```python
from build123d import *

# Parameters (mm, degrees)
F0_R     = 4.75
F1_DEPTH = 7.5
F2_R     = 50
F3_SIZE  = 1
F5_DEPTH = 25
F6_SIZE  = 1


with BuildPart() as f1:
    # F0 (on Top) → F1 (new body, symmetric)
    with BuildSketch(Plane.XY):
        with BuildLine():
            Line((25, 0), (8.288939, 39.506208))
            ThreePointArc((8.288939, 39.506208), (0, 45), (-8.288939, 39.506208))
            Line((-8.288939, 39.506208), (-25, 0))
            Line((-25, 0), (-8.288939, -39.506208))
            ThreePointArc((-8.288939, -39.506208), (0, -45), (8.288939, -39.506208))
            Line((8.288939, -39.506208), (25, 0))
        make_face()
        with Locations((0, -36)):
            Circle(F0_R, mode=Mode.SUBTRACT)
        with Locations((0, 36)):
            Circle(F0_R, mode=Mode.SUBTRACT)
    extrude(amount=F1_DEPTH, both=True)

    # F2
    f2_edges = [f1.edges().sort_by_distance(p)[0] for p in [
        (-25, 0, 0),
        (25, 0, 0),
    ]]
    fillet(f2_edges, radius=F2_R)

    # F3
    f3_edges = [f1.edges().sort_by_distance(p)[0] for p in [
        (0, 45, 7.5),
        (0, 45, -7.5),
        (-12.524692, -29.492569, 7.5),
        (-12.524692, -29.492569, -7.5),
    ]]
    chamfer(f3_edges, length=F3_SIZE)

    # F4 (on face) → F5 (cut)
    with BuildSketch(Plane.XY.offset(7.5)):
        Polygon((-4.025, 6.971505), (-8.05, 0), (-4.025, -6.971505), (4.025, -6.971505), (8.05, 0), (4.025, 6.971505), align=None)
    extrude(amount=-F5_DEPTH, mode=Mode.SUBTRACT)

    # F6
    f6_edges = [f1.edges().sort_by_distance(p)[0] for p in [
        (-4.75, 36, 7.5),
        (-4.75, 36, -7.5),
        (-4.75, -36, 7.5),
        (-4.75, -36, -7.5),
        (0, -6.971505, 7.5),
        (-6.0375, -3.485752, 7.5),
        (-6.0375, 3.485752, 7.5),
        (0, 6.971505, 7.5),
        (6.0375, 3.485752, 7.5),
        (6.0375, -3.485752, 7.5),
        (0, -6.971505, -7.5),
        (6.0375, -3.485752, -7.5),
        (6.0375, 3.485752, -7.5),
        (0, 6.971505, -7.5),
        (-6.0375, 3.485752, -7.5),
    ]]
    chamfer(f6_edges, length=F6_SIZE)


solid = f1.part
```
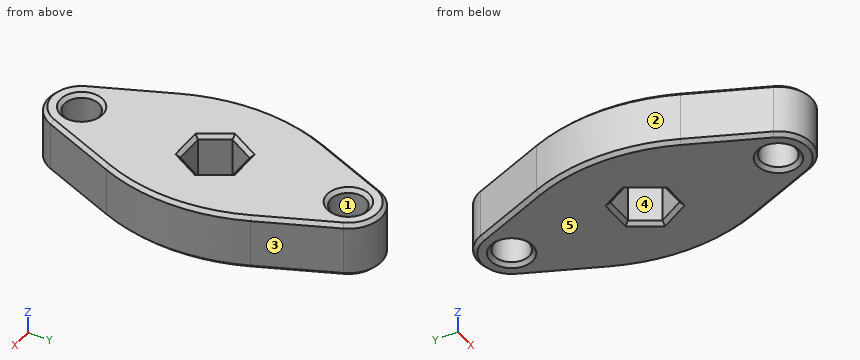
Design review of the part built by this model. Coordinates are the model's own, in mm. Face numbers are marked on the shaded views. A direction names the side the tool comes from. Round coordinates to 2 decimals unless told otherwise and drop trailing zeros. Write each loop counter-clockwise with the first axis right and the second up, starting at its lowest first coordinate (ties: lowest second). Pieces come first, ordered by that corner, then holes.
Item 1: Clearance check with flat-ended pins moving along their axes: pin 1 Ø1.5 at (y, z) = (-7, -5) entering from +X; pin 2 Ø1 at (x, z) = (-0.5, -3) entering from +Y; pin 3 Ø8 at (y, z) = (31.5, 0) entering from -X; pin 4 Ø2 at (y, z) = (33, -1) entering from +X. State where each tip first meets the part, or that it passes through.
Item 2: For probe 1 along Y at (x, z) = (0, 2.5); probe 2 along Y at (x, z) = (-7.5, 4.5); probe 3 along Y at (x, z) = (-7, 6), list the stretches that pass through material, from the lowest coordinate up.
Item 3: We need section A-A on x = 0. State how many separate pieces and enclosed holes the cut face has, and give its area (3 significant figures).
Item 4: For the marked faces 4 and 5, list the 3-axis set-ups (+Z, -Z, +X, -X, +Y, -Y) from which the entire face can be reached by the end or side of a thin tool; tool diameter is ignored.
Item 5: The part is to be moulded in two halves that separate along Y. For the marked faces 1, 2 and 3, say which applies: +Y half, -Y half, draft (parallel to the pull), parting line (faces both ways), or undercut.
Item 6: We need section D-D on y = -25. Write out the cut boundary in (x, z), and give its area (3 significant figures).
Item 7: We need section C-C on y = 36. Write out the cut boundary in (x, z).
Returned:
1. pin 1: stops at x = 20.32
1. pin 2: stops at y = 45
1. pin 3: stops at x = -13.37
1. pin 4: stops at x = 11.46
2. probe 1: y = -45 to -40.75, -31.25 to -6.97, 6.97 to 31.25, 40.75 to 45
2. probe 2: y = -40.97 to -0.95, 0.95 to 40.97
2. probe 3: y = -41.66 to -1.82, 1.82 to 41.66
3. separate pieces: 4
3. enclosed holes: 0
3. area: 848 mm2
4. face 4: +Z, -Z
4. face 5: -Z, +X, -X, +Y, -Y
5. face 1: undercut
5. face 2: parting line
5. face 3: +Y half
6. outline: (-14.43, -6.5) - (-13.34, -7.5) - (13.34, -7.5) - (14.43, -6.5) - (14.43, 6.5) - (13.34, 7.5) - (-13.34, 7.5) - (-14.43, 6.5) - close
6. area: 431 mm2
7. outline: (-9.77, -6.5) - (-8.69, -7.5) - (-5.75, -7.5) - (-4.75, -6.5) - (-4.75, 6.5) - (-5.75, 7.5) - (-8.69, 7.5) - (-9.77, 6.5) - close; (4.75, -6.5) - (5.75, -7.5) - (8.69, -7.5) - (9.77, -6.5) - (9.77, 6.5) - (8.69, 7.5) - (5.75, 7.5) - (4.75, 6.5) - close
